Geometry check sheet. Reference: the model listing, model coordinates, mm. A direction names the side the tool comes from. Give positions to 0.01 mm unless a question says otherwise; leave off trailing zeros. Loops run counter-clockwise (first coordinate to the right, second up) from the corner with the lowest first, then second, coordinate; pieces in that order, holes last. Notation, with made-up numbers: (11, 63) -> (26, 63) arc R21 cw to (26, 79) -> close; hole circle Ø3 at (-39, 68.25). An arc over 180 degrees is marked (long way). Write item = value, one per line.
```python
from build123d import *

# Parameters (mm, degrees)
BOSS_EXTRUDE1_DEPTH = 15
CUT_EXTRUDE1_DEPTH  = 3
BOSS_EXTRUDE2_DEPTH = 5
CUT_EXTRUDE2_DEPTH  = 3
CHAMFER1_SIZE       = 5


with BuildPart() as part:
    # Sketch1 → Boss-Extrude1 (new body)
    with BuildSketch(Plane.XY):
        with BuildLine():
            Line((-55, -13), (-55, 13))
            Line((-55, 13), (-38.445821861, 17.435678664))
            ThreePointArc((-38.445821861, 17.435678664), (-28.606816649, 22.636507401), (-21.999819423, 31.592077218))
            ThreePointArc((-21.999819423, 31.592077218), (0, 46), (21.999819423, 31.592077218))
            ThreePointArc((21.999819423, 31.592077218), (28.606816649, 22.636507401), (38.445821861, 17.435678664))
            Line((38.445821861, 17.435678664), (55, 13))
            Line((55, 13), (55, -13))
            Line((55, -13), (38.445821861, -17.435678664))
            ThreePointArc((38.445821861, -17.435678664), (28.606816649, -22.636507401), (21.999819423, -31.592077218))
            ThreePointArc((21.999819423, -31.592077218), (0, -46), (-21.999819423, -31.592077218))
            ThreePointArc((-21.999819423, -31.592077218), (-28.606816649, -22.636507401), (-38.445821861, -17.435678664))
            Line((-38.445821861, -17.435678664), (-55, -13))
        make_face()
    extrude(amount=BOSS_EXTRUDE1_DEPTH)

    # Sketch2 → Cut-Extrude1 (cut)
    with BuildSketch(Plane.XY.offset(15)):
        with BuildLine():
            Line((36.634088545, -10.67419788), (48, -7.628711084))
            Line((48, -7.628711084), (48, 7.628711084))
            Line((48, 7.628711084), (36.634088545, 10.67419788))
            ThreePointArc((36.634088545, 10.67419788), (24.040161874, 17.331258664), (15.583205424, 28.79438803))
            ThreePointArc((15.583205424, 28.79438803), (0, 39), (-15.583205424, 28.79438803))
            ThreePointArc((-15.583205424, 28.79438803), (-24.040161874, 17.331258664), (-36.634088545, 10.67419788))
            Line((-36.634088545, 10.67419788), (-48, 7.628711084))
            Line((-48, 7.628711084), (-48, -7.628711084))
            Line((-48, -7.628711084), (-36.634088545, -10.67419788))
            ThreePointArc((-36.634088545, -10.67419788), (-24.040161874, -17.331258664), (-15.583205424, -28.79438803))
            ThreePointArc((-15.583205424, -28.79438803), (0, -39), (15.583205424, -28.79438803))
            ThreePointArc((15.583205424, -28.79438803), (24.040161874, -17.331258664), (36.634088545, -10.67419788))
        make_face()
    extrude(amount=-CUT_EXTRUDE1_DEPTH, mode=Mode.SUBTRACT)

    # Sketch3 → Boss-Extrude2 (add)
    with BuildSketch(Plane.XY.offset(12)):
        with BuildLine():
            ThreePointArc((-9.229359568, 14.868386663), (-8.506944444, -15.293197711), (17.5, 0))
            ThreePointArc((17.5, 0), (0, 0), (-9.229359568, 14.868386663))
        make_face()
    extrude(amount=BOSS_EXTRUDE2_DEPTH)

    # Sketch4 → Cut-Extrude2 (cut)
    with BuildSketch(Plane(origin=(0, 0, 0), x_dir=(-1, 0, 0), z_dir=(0, 0, -1))):
        with BuildLine():
            ThreePointArc((-17.5, 0), (0, -17.5), (17.5, 0))
            ThreePointArc((17.5, 0), (15.293197711, 8.506944444), (9.229359568, 14.868386663))
            ThreePointArc((9.229359568, 14.868386663), (0, 0), (-17.5, 0))
        make_face()
    extrude(amount=-CUT_EXTRUDE2_DEPTH, mode=Mode.SUBTRACT)

    # Chamfer1
    chamfer1_edges = [part.edges().sort_by_distance(p)[0] for p in [
        (55, -13, 7.5),
        (55, 13, 7.5),
        (-55, 13, 7.5),
        (-55, -13, 7.5),
    ]]
    chamfer(chamfer1_edges, length=CHAMFER1_SIZE)


solid = part.part
```
Item 1: Draft check along X on faces 3 (the flat face through (-42.4, -9.13, 13.52)), 4 (the flat face through (1, 1, 0)), 5 (the cylindrical face through (-28.73, 22.53, 7.4)). Enter one of: +X half, -X half, draft (parallel to the pull), parting line (faces both ways), or undercut.
Answer:
face_3 = undercut
face_4 = draft
face_5 = -X half
Item 2: Section check C-C, the plane y = -23. Record the cut outline in (x, z), plus the area to 3 significant figures.
Answer:
outline = (-28.19, 0) -> (28.19, 0) -> (28.19, 15) -> (18.87, 15) -> (18.87, 12) -> (-18.87, 12) -> (-18.87, 15) -> (-28.19, 15) -> close
area = 733 mm^2
Item 3: Tool access check on faces 1 (the cylindrical face through (0, 46, 7)), 2 (the flat face through (48, 0, 14)). Record the directions out of +Z, -Z, +X, -X, +Y, -Y that give a thin tool (end or side, any length) a straight path to the whole face; none if there is none.
Answer:
face_1 = +Z, -Z, +Y
face_2 = +Z
Item 4: Thickness scan on L1, parallel to X at y = 3, z = 12.5; L2, parallel to Y at x = 18, z = 13; L3, parallel to Z at x = 2, y = 36.5. Record the ranges inside material, lowest first. Write a range as [from, to].
Answer:
L1 = [-55, -48], [-17.24, -3.98], [48, 55]
L2 = [-37.87, -24.28], [24.28, 37.87]
L3 = [0, 12]
Item 5: Section check B-B, the plane z = 6.25. Record the cut outline in (x, y), plus the area to 3 significant figures.
Answer:
outline = (-55, -8) -> (-50.17, -14.29) -> (-38.45, -17.44) arc R25 cw to (-22, -31.59) arc R24 ccw to (22, -31.59) arc R25 cw to (38.45, -17.44) -> (50.17, -14.29) -> (55, -8) -> (55, 8) -> (50.17, 14.29) -> (38.45, 17.44) arc R25 cw to (22, 31.59) arc R24 ccw to (-22, 31.59) arc R25 cw to (-38.45, 17.44) -> (-50.17, 14.29) -> (-55, 8) -> close
area = 6,120 mm^2
Item 6: Gauge pin test, flat ends, axial feed: pin 1 (6 mm diameter, centred on y = 35, z = 7.5, fed in from -X); pin 2 (1 mm diameter, centred on x = 19.5, z = 3, fed in from -Y); pin 3 (1.5 mm diameter, centred on y = 12, z = 3, fed in from +X). Record the tip position at first contact, or that the pin passes through.
Answer:
pin_1 = -21.82
pin_2 = -36.66
pin_3 = 52.51
Item 7: Section check A-A, the plane x = 0. Record the cut outline in (y, z).
Answer:
outline = (-46, 0) -> (-17.5, 0) -> (-17.5, 3) -> (0, 3) -> (0, 0) -> (46, 0) -> (46, 15) -> (39, 15) -> (39, 12) -> (0, 12) -> (0, 17) -> (-17.5, 17) -> (-17.5, 12) -> (-39, 12) -> (-39, 15) -> (-46, 15) -> close
Item 8: Section check D-D, the plane x = 31. Record the cut outline in (y, z).
Answer:
outline = (-20.82, 0) -> (20.82, 0) -> (20.82, 15) -> (12.77, 15) -> (12.77, 12) -> (-12.77, 12) -> (-12.77, 15) -> (-20.82, 15) -> close
